Read the model definition and answer for the solid it produces. Units are mm, in the model's axes. Face numbers are marked on the shaded views. A direction names the side the tool comes from. Give positions to 0.01 mm unless a question says otherwise; leave off trailing zeros. Write each loop counter-clockwise with the first axis right and the second up, starting at its lowest first coordinate (ties: lowest second). Pieces come first, ordered by that corner, then holes. Notation, with made-up numbers: M -21.75,-12 L 18.25,-12 A20 cw 18.25,9 Z; hole C -20.75,-10 d6. An arc over 180 degrees is marked long. Put each result on its own line as item: value.
Solid Edge part; units mm, degrees
sketch "Sketch1" plane through (0, 0, 0) normal (0, 0, 1) x (1, 0, 0)
  line L0 (0, 0) -> (30, 0)
  line L1 (30, 0) -> (30, 10)
  line L2 (30, 10) -> (40, 10)
  line L3 (40, 10) -> (40, 0)
  line L4 (40, 0) -> (61.2132, -21.2132)
  line L5 (51.2132, -31.2132) -> (61.2132, -21.2132)
  line L6 (30, -10) -> (51.2132, -31.2132)
  line L7 (0, -10) -> (30, -10)
  line L8 (0, 0) -> (0, -10)
extrude "Protrusion1" add sketch "Sketch1" along normal blind 60
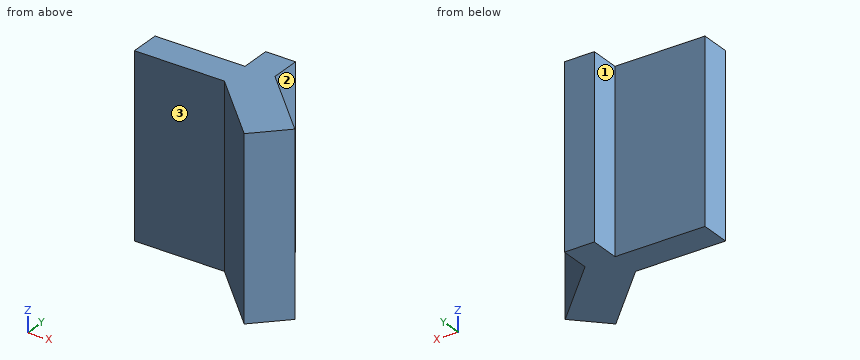
(1) Section A-A on z = 10 is taken. Determine the outline of the cut face in (x, y), and give its area (3 significant figures).
Result:
outline: M 0,-10 L 30,-10 L 51.21,-31.21 L 61.21,-21.21 L 40,0 L 40,10 L 30,10 L 30,0 L 0,0 Z
area: 874 mm²
(2) Section C-C on y = 6 is taken. Determine the outline of the cut face in (x, z), and give its area (3 significant figures).
Result:
outline: M 30,0 L 40,0 L 40,60 L 30,60 Z
area: 600 mm²
(3) Section B-B on x = 7 is taken. Determine the outline of the cut face in (y, z).
Result:
outline: M -10,0 L 0,0 L 0,60 L -10,60 Z
(4) Given pin 1 Ø24 at (x, z) = (15, 42.5) entering from -Y; pin 2 Ø9 at (x, z) = (8.5, 23.5) entering from +Y; pin 3 Ø2 at (y, z) = (2.5, 31.5) entering from -X, each flat-ended and moving along its own axis, determine where each tip first touches the part or whether it passes through.
Result:
pin 1: stops at y = -10
pin 2: stops at y = 0
pin 3: stops at x = 30
(5) Which of the six approach directions +Z, -Z, +X, -X, +Y, -Y give full straight-line access (tool end or side, diameter ignored) to the marked faces 1, 2 and 3?
Result:
face 1: +Z, -Z, -X, +Y
face 2: +Z, -Z, +X, +Y
face 3: +Z, -Z, -X, -Y
(6) Straight lines are drawn through the part: line 1 along Y through (x, z) = (9, 29.5); line 2 along X through (y, z) = (3.5, 33); line 3 along X through (y, z) = (-12.5, 34). For each, find the intervals that lie inside material, in ascending order. Write a range as from..to.
Result:
line 1: y = -10..0
line 2: x = 30..40
line 3: x = 32.5..52.5
